Verification items for this drawing (mm, ordinates from the low corner). Round coordinates to 2 decimals unless told otherwise and drop trailing zeros. Order: outer loops, then holes, each group sorted by start corner. A loop starts at its lowest first (then second) coordinate and runs counter-clockwise, first axis right, second up. Notation, with made-up numbers: (7.5, 38) - (47.5, 38) arc R6 ccw to (47.5, 43) - close; hole circle Ø11 at (17.5, 33). An arc over 180 degrees is marked (long way). Return JSON: item names as keys, results as strings. Group by question number.
Q1. Sectioned sample at A-A, the plane y = 66.04. Record the cut outline in (x, z) (3 decimals).
Q2. Material ranges on line 1 along Y through (x, z) = (29.21, 3.5) (3 decimals); line 2 along Y through (x, z) = (31, 2.5); line 3 along Y through (x, z) = (19, 6.25), recorded low to high.
Q3. Sectioned sample at D-D, the plane x = 17. Record the cut outline in (y, z), then the cut area to 3 significant figures.
Q4. Sectioned sample at B-B, the plane z = 2. Record the cut outline in (x, y) (3 decimals), then the cut area to 3 significant figures.
Q5. Sectioned sample at C-C, the plane x = 29.5. Record the cut outline in (y, z), then the cut area to 3 significant figures.
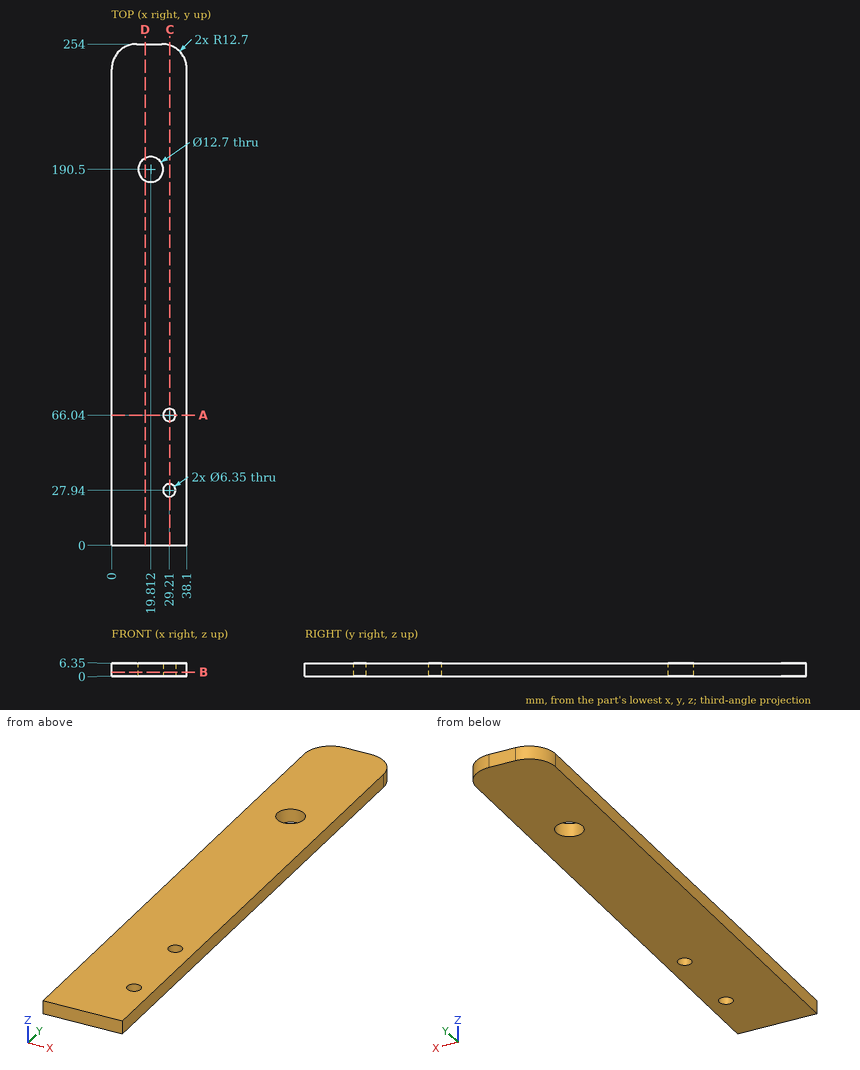
Reply:
{
 "1": {"outline": "(0, 0) - (26.035, 0) - (26.035, 6.35) - (0, 6.35) - close; (32.385, 0) - (38.1, 0) - (38.1, 6.35) - (32.385, 6.35) - close"},
 "2": {"line 1": "0 to 24.765, 31.115 to 62.865, 69.215 to 253.415", "line 2": "0 to 25.32, 30.56 to 63.42, 68.66 to 252.7", "line 3": "0 to 184.2, 196.8 to 254"},
 "3": {"outline": "(0, 0) - (184.81, 0) - (184.81, 6.35) - (0, 6.35) - close; (196.19, 0) - (254, 0) - (254, 6.35) - (196.19, 6.35) - close", "area": "1,540 mm^2"},
 "4": {"outline": "(0, 0) - (38.1, 0) - (38.1, 241.3) arc R12.7 ccw to (25.4, 254) - (12.7, 254) arc R12.7 ccw to (0, 241.3) - close; hole circle Ø12.7 at (19.812, 190.5); hole circle Ø6.35 at (29.21, 27.94); hole circle Ø6.35 at (29.21, 66.04)", "area": "9,420 mm^2"},
 "5": {"outline": "(0, 0) - (24.78, 0) - (24.78, 6.35) - (0, 6.35) - close; (31.1, 0) - (62.88, 0) - (62.88, 6.35) - (31.1, 6.35) - close; (69.2, 0) - (253.32, 0) - (253.32, 6.35) - (69.2, 6.35) - close", "area": "1,530 mm^2"}
}
